```python
from build123d import *

# Parameters (mm, degrees)
PAD001_DEPTH = 1.75
SKETCH002_R  = 2.3
PAD002_DEPTH = 6.5
SKETCH_R     = 5.9
PAD_DEPTH    = 6
SKETCH003_R  = 6.5
PAD003_DEPTH = 0.6


with BuildPart() as pad001:
    # Sketch001 → Pad001 (new body, symmetric)
    with BuildSketch(Plane.XZ):
        Polygon((3.525, -2.03516), (3.525, 2.03516), (0, 4.070319), (-3.525, 2.03516), (-3.525, -2.03516), (-3.525, -6), (3.525, -6), align=None)
    extrude(amount=PAD001_DEPTH, both=True)


with BuildPart() as pad002:
    # Sketch002 → Pad002 (new body, symmetric)
    with BuildSketch(Plane.XZ):
        Circle(SKETCH002_R)
    extrude(amount=PAD002_DEPTH, both=True)


with BuildPart() as pad003:
    # Sketch → Pad (new body, symmetric)
    with BuildSketch(Plane.XY):
        Circle(SKETCH_R)
    extrude(amount=PAD_DEPTH, both=True)

    # Cut: cut Pad002
    add(pad002.part, mode=Mode.SUBTRACT)

    # Cut001: cut Pad001
    add(pad001.part, mode=Mode.SUBTRACT)

    # Sketch003 → Pad003 (new body)
    with BuildSketch(Plane.XY.offset(6)):
        Circle(SKETCH003_R)
    extrude(amount=PAD003_DEPTH)


solid = pad003.part
```
Source: CAD feature listing. Evaluate the final solid. Frame: model axes, mm. A direction names the side the tool comes from. Coordinates: 2 decimals unless noted, no trailing zeros. Loops run counter-clockwise (first coordinate to the right, second up) from the corner with the lowest first, then second, coordinate; pieces in that order, holes last. Notation, with made-up numbers: M 6,-22 L 63,-22 A4 cw 63,-17 Z; hole C 86.25,12 d3. An arc over 180 degrees is marked long. Put each result on its own line as item: value. Start each with the question number.
1) Cut plane D-D on y = 0. Return the cut outline in (x, z) (3 decimals).
2) Reachability of faces 1 (the face through (0, -3, -6)), 2 (the face through (5.45, -2.26, 0.08)) from +Z, -Z, +X, -X, +Y, -Y: full face, straight path, thin tool, end or side. Return the list, or none.
3) Cut plane B-B on y = -3.5. Return the cut outline in (x, z).
4) Contact query for flat-ended pins moving along their axis: pin 1 Ø1 at (y, z) = (-0.5, 1) entering from -X; pin 2 Ø3.5 at (x, z) = (1, -0.5) entering from +Y; pin 3 Ø1 at (x, z) = (-0.5, 2.5) entering from -Y. Output: stop coordinate, or through.
5) Cut plane C-C on x = -1. Return the cut outline in (y, z).
6) Cut plane A-A on z = 0. Return the cut outline in (x, y) (3 decimals).
7) Ray query, L1, parallel to Z at x = 0, y = 3.35; L2, parallel to Z at x = 5.25, y = 3.5; L3, parallel to Z at x = -1.25, y = 3.5. Return the intervals inside material, ascending. Write a range as from..to.
8) Pull-direction query (X, two-part tool) for faces 3 (the face through (1, -6, 6)), 4 (the face through (-5.158, -3.955, 6.296)), 5 (the face through (-0.3, 3.8, 2.28)); classes: pulls with the +X half, pulls with the -X half, needs draft (parallel to the pull), parting line crosses it, or undercut.
The answers:
1. outline: M -6.5,6 L -5.9,6 L -5.9,-6 L -3.525,-6 L -3.525,2.035 L 0,4.07 L 3.525,2.035 L 3.525,-6 L 5.9,-6 L 5.9,6 L 6.5,6 L 6.5,6.6 L -6.5,6.6 Z
2. face 1: -Z, +X, -X, +Y, -Y
2. face 2: -Z
3. outline: M -5.48,6 L -4.75,6 L -4.75,-6 L 4.75,-6 L 4.75,6 L 5.48,6 L 5.48,6.6 L -5.48,6.6 Z; hole C 0,0 d4.6
4. pin 1: stops at x = -5.9
4. pin 2: stops at y = 5.87
4. pin 3: stops at y = -5.9
5. outline: M -6.42,6 L -5.81,6 L -5.81,2.07 L -1.75,2.07 L -1.75,3.49 L 1.75,3.49 L 1.75,2.07 L 5.81,2.07 L 5.81,6 L 6.42,6 L 6.42,6.6 L -6.42,6.6 Z; M -5.81,-6 L -1.75,-6 L -1.75,-2.07 L -5.81,-2.07 Z; M 1.75,-6 L 5.81,-6 L 5.81,-2.07 L 1.75,-2.07 Z
6. outline: M -3.525,-1.75 L -3.525,1.75 L -2.3,1.75 L -2.3,5.433 A5.9 ccw -2.3,-5.433 L -2.3,-1.75 Z; M 2.3,-5.433 A5.9 ccw 2.3,5.433 L 2.3,1.75 L 3.525,1.75 L 3.525,-1.75 L 2.3,-1.75 Z
7. L1: z = -6..-2.3, 2.3..6.6
7. L2: z = 6..6.6
7. L3: z = -6..-1.93, 1.93..6.6
8. face 3: needs draft
8. face 4: parting line crosses it
8. face 5: undercut
